Check sheet for the modelled part. Datum: model origin and axes. Units: mm. A direction names the side the tool comes from. Coordinates: 2 decimals unless noted, no trailing zeros. Write each loop counter-clockwise with the first axis right and the second up, starting at its lowest first coordinate (ties: lowest second). Pieces come first, ordered by that corner, then holes. Notation, with made-up numbers: M -31,37.25 L -13,37.25 A31 ccw -13,62.25 Z; hole C 65,56 d5. An arc over 180 degrees is marked long. Answer as CSV lines item,"result". Start each with the question number.
1) Section check D-D (x = 52). Record the cut outline in (y, z) (3 decimals), and give its area (3 significant figures).
2) Section check A-A (y = 28). Record the cut outline in (x, z) (3 decimals), and give its area (3 significant figures).
3) Section check C-C (y = 10.5). Record the cut outline in (x, z) (3 decimals), and give its area (3 significant figures).
4) Access from +Z, -Z, +X, -X, +Y, -Y to the whole of each face (thin tool, end or side, straight path). Record for faces 5 (the flat face through (0, -63.5, 0)), 6 (the cylindrical face through (-39.464, 61.59, -0.133)), 7 (the flat face through (41.275, -1, 4)), 8 (the flat face through (22.225, 17, 18)), 9 (the flat face through (-6, -7.938, 30)).
5) Draft check along X on faces 1 (the cylindrical face through (39.464, 61.59, 0.133)), 2 (the flat face through (-41.275, -1, 0)), 3 (the flat face through (79, 0, 66.675)), 4 (the cylindrical face through (44.047, -0.356, 35.962)). Enter one of: +X half, -X half, draft (parallel to the pull), parting line (faces both ways), or undercut.
6) Section check B-B (z = -2). Record the cut outline in (x, y) (3 decimals), and give its area (3 significant figures).
7) Material ranges on L1, parallel to X at y = 15.5, z = -2 (3 decimals); L2, parallel to Z at x = -11, y = 35.5 (3 decimals); L3, parallel to X at y = 23.5, z = 16 (3 decimals), recorded low to high. Write a range as [from, to].
8) Go/stop test with flat-tipped pins: pin 1 Ø2 at (x, z) = (45, 40.5) entering from +Y; pin 2 Ø5 at (y, z) = (5, 37.5) entering from +X; pin 3 Ø5 at (y, z) = (19.5, 19) entering from -X (3 decimals). Record where each tip stops, or that it passes through.
from build123d import *

# Parameters (mm, degrees)
F1_DEPTH = 63.5
F0_W     = 18.940978
F0_H     = 4.7752
F2_DEPTH = 25.4
F3_DEPTH = 7.9375
F5_R     = 6.35


with BuildPart() as f1:
    # F0 (on Front) → F1 (new body, symmetric)
    with BuildSketch(Plane.XZ):
        Polygon((22.225, 9.525), (-41.275, 9.525), (-41.275, -9.525), (41.275, -9.525), (41.275, 9.525), align=None)
    extrude(amount=F1_DEPTH, both=True)

    # F0 (on Front) → F2 (join, symmetric)
    with BuildSketch(Plane.XZ):
        with BuildLine():
            Line((22.225, 27.0002), (22.225, 9.525))
            Line((22.225, 9.525), (41.275, 9.525))
            Line((41.275, 9.525), (41.275, 27.0002))
            ThreePointArc((41.275, 27.0002), (45.92468, 38.22552), (57.15, 42.8752))
            Line((57.15, 42.8752), (60.325, 42.8752))
            Line((60.325, 42.8752), (60.325, 61.9252))
            Line((60.325, 61.9252), (57.15, 61.9252))
            add(Edge.make_bspline(
                [(53.775986, 61.761841), (54.917226, 61.840319), (56.042547, 61.89509), (57.15, 61.9252)],
                knots=[108.292416, 108.292416, 108.292416, 108.292416, 111.504536, 111.504536, 111.504536, 111.504536], degree=3))
            ThreePointArc((53.775986, 61.761841), (31.288899, 50.472718), (22.225, 27.0002))
        make_face()
        with Locations((69.795489, 40.4876)):
            Rectangle(F0_W, F0_H)
    extrude(amount=F2_DEPTH, both=True)

    # F0 (on Front) → F3 (join, symmetric)
    with BuildSketch(Plane.XZ):
        with BuildLine():
            add(Edge.make_bspline(
                [(-41.275, 9.525), (-41.269137, 29.523659), (15.30057, 59.116032), (53.775986, 61.761841)],
                knots=[0, 0, 0, 0, 108.292416, 108.292416, 108.292416, 108.292416], degree=3))
            Line((-41.275, 9.525), (22.225, 9.525))
            Line((22.225, 9.525), (22.225, 27.0002))
            ThreePointArc((22.225, 27.0002), (31.288899, 50.472718), (53.775986, 61.761841))
        make_face()
    extrude(amount=F3_DEPTH, both=True)

    # F0 (on Front) → F4 (revolve)
    with BuildSketch(Plane.XZ):
        Polygon((79.265978, 66.675), (79.265978, 61.9252), (79.265978, 49.505379), (79.265978, 42.8752), (79.265978, 38.1), (111.125, 38.1), (111.125, 66.675), align=None)
    revolve(axis=Axis((79.265978, 0, 52.3875), (0, 0, -1)))

    # F5
    f5_edges = [f1.edges().sort_by_distance(p)[0] for p in [
        (41.275, -63.5, 0),
        (-41.275, -63.5, 0),
        (41.275, 63.5, 0),
        (-41.275, 63.5, 0),
    ]]
    fillet(f5_edges, radius=F5_R)


solid = f1.part
Results found:
1,outline,"M -25.4,42.017 L -16.479,42.017 L -16.479,38.1 L 16.479,38.1 L 16.479,42.017 L 25.4,42.017 L 25.4,61.543 L 16.479,61.543 L 16.479,66.675 L -16.479,66.675 L -16.479,61.543 L -25.4,61.543 Z"
1,area,"1,290 mm2"
2,outline,"M -41.275,-9.525 L 41.275,-9.525 L 41.275,9.525 L -41.275,9.525 Z; M 64.067,38.1 L 94.465,38.1 L 94.465,66.675 L 64.067,66.675 Z"
2,area,"2,440 mm2"
3,outline,"M -41.275,-9.525 L 41.275,-9.525 L 41.275,27 A15.875 cw 49.187,40.734 L 49.187,38.1 L 109.345,38.1 L 109.345,66.675 L 49.187,66.675 L 49.187,61.005 A34.925 ccw 22.225,27 L 22.225,9.525 L -41.275,9.525 Z"
3,area,"4,230 mm2"
4,face 5,"+Z, -Z, +X, -X, -Y"
4,face 6,"+Z, -Z, -X, +Y"
4,face 7,"-Z, +X, +Y, -Y"
4,face 8,"+Z, -X, +Y"
4,face 9,"+Z, -X, -Y"
5,face 1,"+X half"
5,face 2,"-X half"
5,face 3,"draft"
5,face 4,"undercut"
6,outline,"M -41.275,-57.15 A6.35 ccw -34.925,-63.5 L 34.925,-63.5 A6.35 ccw 41.275,-57.15 L 41.275,57.15 A6.35 ccw 34.925,63.5 L -34.925,63.5 A6.35 ccw -41.275,57.15 Z"
6,area,"10,400 mm2"
7,L1,"x = [-41.275, 41.275]"
7,L2,"z = [-9.525, 9.525]"
7,L3,"x = [22.225, 41.275]"
8,pin 1,"stops at y = 25.4"
8,pin 2,"stops at x = 111.02"
8,pin 3,"stops at x = 22.225"
